```python
from build123d import *

# Parameters (mm, degrees)
SKETCH1_W                       = 30
SKETCH1_H                       = 40
BOSS_EXTRUDE1_DEPTH             = 3
TAP_DRILL_FOR_M3_TAP1_OUTLINE_R = 1.25
TAP_DRILL_FOR_M3_TAP1_DEPTH     = 3
TAP_DRILL_FOR_M8_TAP1_D         = 6.8
TAP_DRILL_FOR_M8_TAP1_DEPTH     = 3


# Read off the part's stored shape, not the designer's step: Tap Drill for M3 Tap1
with BuildPart() as part:
    # Sketch1 → Boss-Extrude1 (new body)
    with BuildSketch(Plane.XY):
        with Locations((15, 20)):
            Rectangle(SKETCH1_W, SKETCH1_H)
    extrude(amount=BOSS_EXTRUDE1_DEPTH)

    # Tap Drill for M3 Tap1 outline → Tap Drill for M3 Tap1 (cut)
    with BuildSketch(Plane.XY):
        with Locations((25, 6)):
            Circle(TAP_DRILL_FOR_M3_TAP1_OUTLINE_R)
        with Locations((5, 34)):
            Circle(TAP_DRILL_FOR_M3_TAP1_OUTLINE_R)
        with Locations((5, 6)):
            Circle(TAP_DRILL_FOR_M3_TAP1_OUTLINE_R)
        with Locations((25, 34)):
            Circle(TAP_DRILL_FOR_M3_TAP1_OUTLINE_R)
        with Locations((15, 20)):
            Circle(TAP_DRILL_FOR_M3_TAP1_OUTLINE_R)
    extrude(amount=TAP_DRILL_FOR_M3_TAP1_DEPTH, mode=Mode.SUBTRACT)

    # Tap Drill for M8 Tap1
    with Locations(Plane.XY.offset(3)):
        with Locations((15, 20)):
            Hole(TAP_DRILL_FOR_M8_TAP1_D / 2, depth=TAP_DRILL_FOR_M8_TAP1_DEPTH)


solid = part.part
```
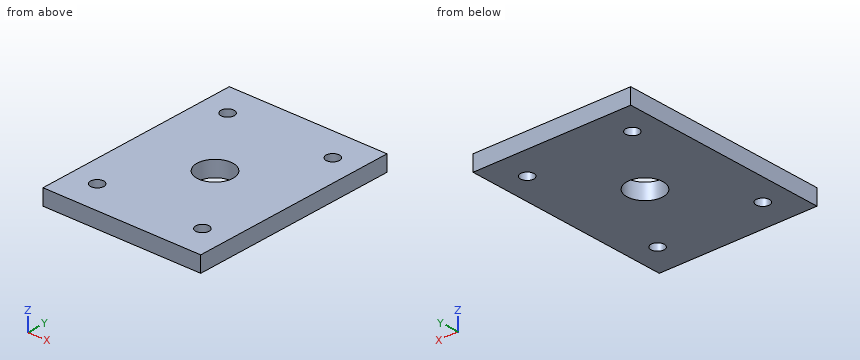
Here's how the part is built. I have some questions about the finished solid (model axes, mm). Round coordinates to 2 decimals unless told otherwise and drop trailing zeros. Loops run counter-clockwise (first coordinate to the right, second up) from the corner with the lowest first, then second, coordinate; pieces in that order, holes last. Notation, with made-up numbers: (43, 79.25) -> (73, 79.25) arc R10 cw to (73, 95.25) -> close; hole circle Ø2 at (58, 43.5). An arc over 180 degrees is marked (long way). Answer as CSV lines item,"result". Start each with the question number.
1. Imagine slicing it at D-D on y = 21. Write out the boundary of the cut face in (x, z), plus the area to 3 significant figures.
2. Imagine slicing it at B-B on y = 6. Write out the boundary of the cut face in (x, z), plus the area to 3 significant figures.
3. Imagine slicing it at C-C on x = 15. Write out the boundary of the cut face in (y, z), plus the area to 3 significant figures.
4. I need wall thicknesses on probe 1 along Y at (x, z) = (25, 2); probe 2 along Y at (x, z) = (4, 1.8); probe 3 along X at (y, z) = (5.5, 1.55). Which ranges of each line are inside material? Lowest first, please. Write a range as from..to.
5. Imagine slicing it at A-A on z = 1.45. Write out the boundary of the cut face in (x, y), plus the area to 3 significant figures.
Solution:
1,outline,"(0, 0) -> (11.75, 0) -> (11.75, 3) -> (0, 3) -> close; (18.25, 0) -> (30, 0) -> (30, 3) -> (18.25, 3) -> close"
1,area,"70.5 mm²"
2,outline,"(0, 0) -> (3.75, 0) -> (3.75, 3) -> (0, 3) -> close; (6.25, 0) -> (23.75, 0) -> (23.75, 3) -> (6.25, 3) -> close; (26.25, 0) -> (30, 0) -> (30, 3) -> (26.25, 3) -> close"
2,area,"75.0 mm²"
3,outline,"(0, 0) -> (16.6, 0) -> (16.6, 3) -> (0, 3) -> close; (23.4, 0) -> (40, 0) -> (40, 3) -> (23.4, 3) -> close"
3,area,"99.6 mm²"
4,probe 1,"0..4.75, 7.25..32.75, 35.25..40"
4,probe 2,"0..5.25, 6.75..33.25, 34.75..40"
4,probe 3,"0..3.85, 6.15..23.85, 26.15..30"
5,outline,"(0, 0) -> (30, 0) -> (30, 40) -> (0, 40) -> close; hole circle Ø2.5 at (5, 6); hole circle Ø2.5 at (5, 34); hole circle Ø6.8 at (15, 20); hole circle Ø2.5 at (25, 6); hole circle Ø2.5 at (25, 34)"
5,area,"1,140 mm²"
